Answer from the drawing. Dimensions are ordinates in mm from the lowest x, y and z of the part. Coordinates: 2 decimals unless noted, no trailing zeros. Loops run counter-clockwise (first coordinate to the right, second up) from the corner with the lowest first, then second, coordinate; pieces in that order, holes last.
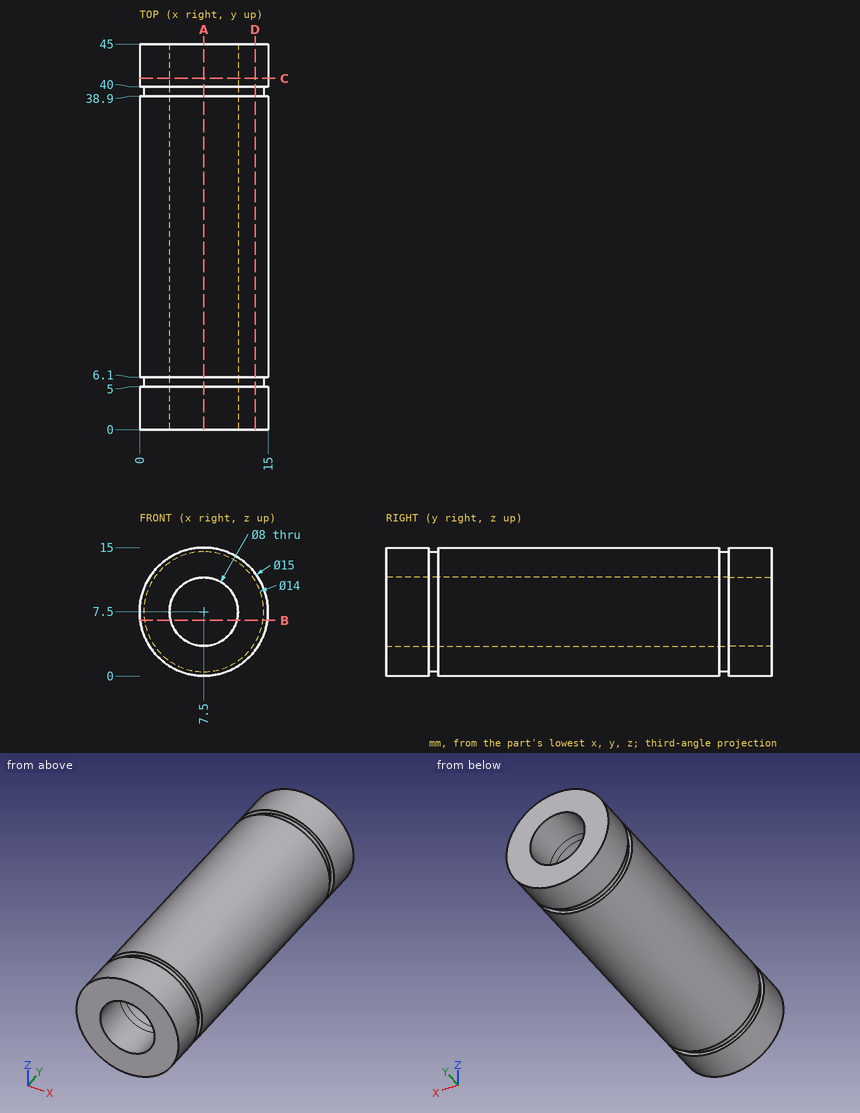
Item 1: A cutting plane is placed at A-A on x = 7.5. Determine the outline of the cut face in (y, z).
Numbers:
outline: (0, 0) - (5, 0) - (5, 0.5) - (6.1, 0.5) - (6.1, 0) - (38.9, 0) - (38.9, 0.5) - (40, 0.5) - (40, 0) - (45, 0) - (45, 3.5) - (0, 3.5) - close; (0, 11.5) - (45, 11.5) - (45, 15) - (40, 15) - (40, 14.5) - (38.9, 14.5) - (38.9, 15) - (6.1, 15) - (6.1, 14.5) - (5, 14.5) - (5, 15) - (0, 15) - close
Item 2: Find the intervals of material crossed by line 1 along X through (y, z) = (14, 7.5); line 2 along Y through (x, z) = (10.75, 13.75); line 3 along X through (y, z) = (39.5, 7.5), in increasing order.
Numbers:
line 1: x = 0 to 3.5, 11.5 to 15
line 2: y = 0 to 5, 6.1 to 38.9, 40 to 45
line 3: x = 0.5 to 3.5, 11.5 to 14.5
Item 3: A cutting plane is placed at C-C on y = 41. Determine the outline of the cut face in (x, z).
Numbers:
outline: circle Ø15 at (7.5, 7.5); hole circle Ø8 at (7.5, 7.5)
Item 4: A cutting plane is placed at D-D on x = 13.5. Determine the outline of the cut face in (y, z).
Numbers:
outline: (0, 3) - (5, 3) - (5, 3.89) - (6.1, 3.89) - (6.1, 3) - (38.9, 3) - (38.9, 3.89) - (40, 3.89) - (40, 3) - (45, 3) - (45, 12) - (40, 12) - (40, 11.11) - (38.9, 11.11) - (38.9, 12) - (6.1, 12) - (6.1, 11.11) - (5, 11.11) - (5, 12) - (0, 12) - close
Item 5: A cutting plane is placed at B-B on z = 6.5. Determine the outline of the cut face in (x, y), then the cut area to 3 significant figures.
Numbers:
outline: (0.07, 0) - (3.63, 0) - (3.63, 45) - (0.07, 45) - (0.07, 40) - (0.57, 40) - (0.57, 38.9) - (0.07, 38.9) - (0.07, 6.1) - (0.57, 6.1) - (0.57, 5) - (0.07, 5) - close; (11.37, 0) - (14.93, 0) - (14.93, 5) - (14.43, 5) - (14.43, 6.1) - (14.93, 6.1) - (14.93, 38.9) - (14.43, 38.9) - (14.43, 40) - (14.93, 40) - (14.93, 45) - (11.37, 45) - close
area: 318 mm2
Item 6: Given pin 1 (7 mm diameter, centred on x = 7.5, z = 7.5, fed in from +Y); pin 2 (6 mm diameter, centred on y = 8.5, z = 12, fed in from -X); pin 3 (1 mm diameter, centred on y = 33.5, z = 13.5, fed in from -X); pin 4 (2 mm diameter, centred on x = 11, y = 34, fed in from +Z), each flat-ended and moving along its own axis, determine where each tip first touches the part or whether it passes through.
Numbers:
pin 1: passes through
pin 2: stops at x = 0.15
pin 3: stops at x = 2.4
pin 4: stops at z = 14.57
